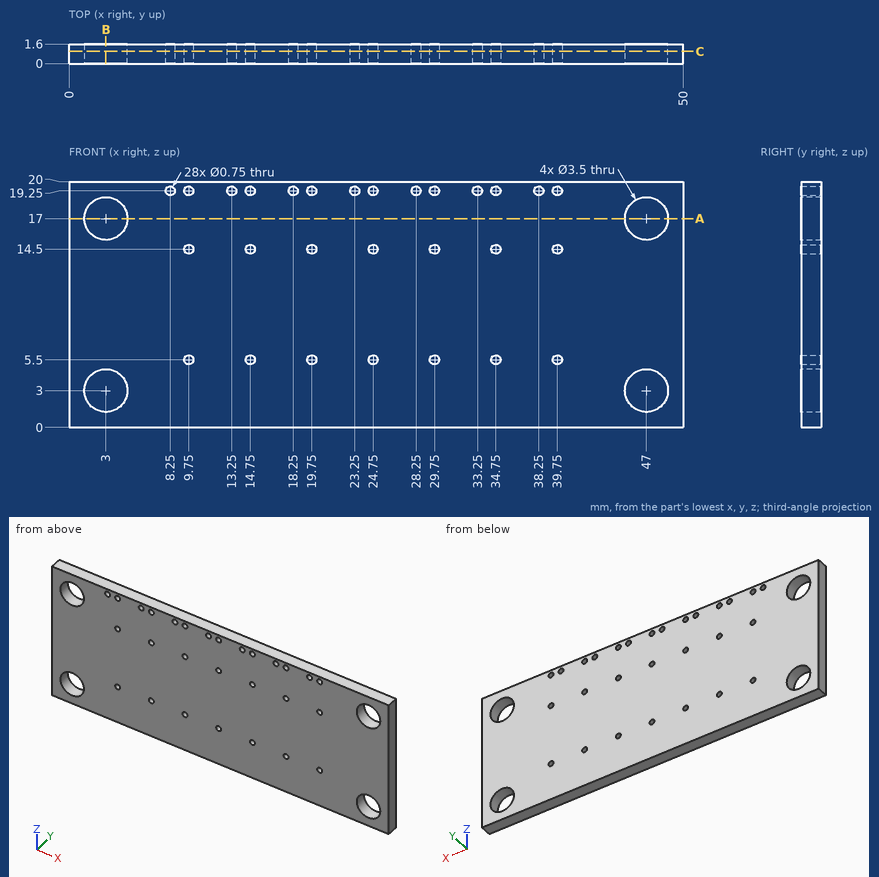
Job drawing, mm, ordinate dimensions from the low corner. One solid piece. Coordinates: 2 decimals unless noted, no trailing zeros. Loops run counter-clockwise (first coordinate to the right, second up) from the corner with the lowest first, then second, coordinate; pieces in that order, holes last. Notation, with made-up numbers: (68, 46.5) - (77, 46.5) arc R23 ccw to (77, 65.5) - close; hole circle Ø11 at (20, 89.5). An arc over 180 degrees is marked (long way). Answer as a JSON object with one key per item and string values. Group by question number.
(1) Cut at A-A (z = 17). Give the cut face in (x, y).
(2) Cut at B-B (x = 3). Give the cut face in (y, z), then the cut area to 3 significant figures.
(3) Cut at C-C (y = 1). State how many separate pieces and enclosed holes the cut face has, then the cut area to 3 significant figures.
(4) Flat gauge pin, fed straight in: pin 1 (4 mm diameter, centred on x = 42.5, z = 2.5, fed in from -Y). Where does the tip first touch, or does it go through?
(5) Probe line 1 along Z through (x, y) = (19.75, 1.1) (3 decimals); line 2 along X through (y, z) = (0.9, 17); line 3 along Z through (x, y) = (18.25, 0.5) (3 decimals). List the from-to ranges inside material, lowest first.
Geometry says:
{
 "1": {"outline": "(0, 0) - (1.25, 0) - (1.25, 1.6) - (0, 1.6) - close; (4.75, 0) - (45.25, 0) - (45.25, 1.6) - (4.75, 1.6) - close; (48.75, 0) - (50, 0) - (50, 1.6) - (48.75, 1.6) - close"},
 "2": {"outline": "(0, 0) - (1.6, 0) - (1.6, 1.25) - (0, 1.25) - close; (0, 4.75) - (1.6, 4.75) - (1.6, 15.25) - (0, 15.25) - close; (0, 18.75) - (1.6, 18.75) - (1.6, 20) - (0, 20) - close", "area": "20.8 mm^2"},
 "3": {"separate pieces": "1", "enclosed holes": "32", "area": "949 mm^2"},
 "4": {"pin 1": "stops at y = 0"},
 "5": {"line 1": "z = 0 to 5.125, 5.875 to 14.125, 14.875 to 18.875, 19.625 to 20", "line 2": "x = 0 to 1.25, 4.75 to 45.25, 48.75 to 50", "line 3": "z = 0 to 18.875, 19.625 to 20"}
}
